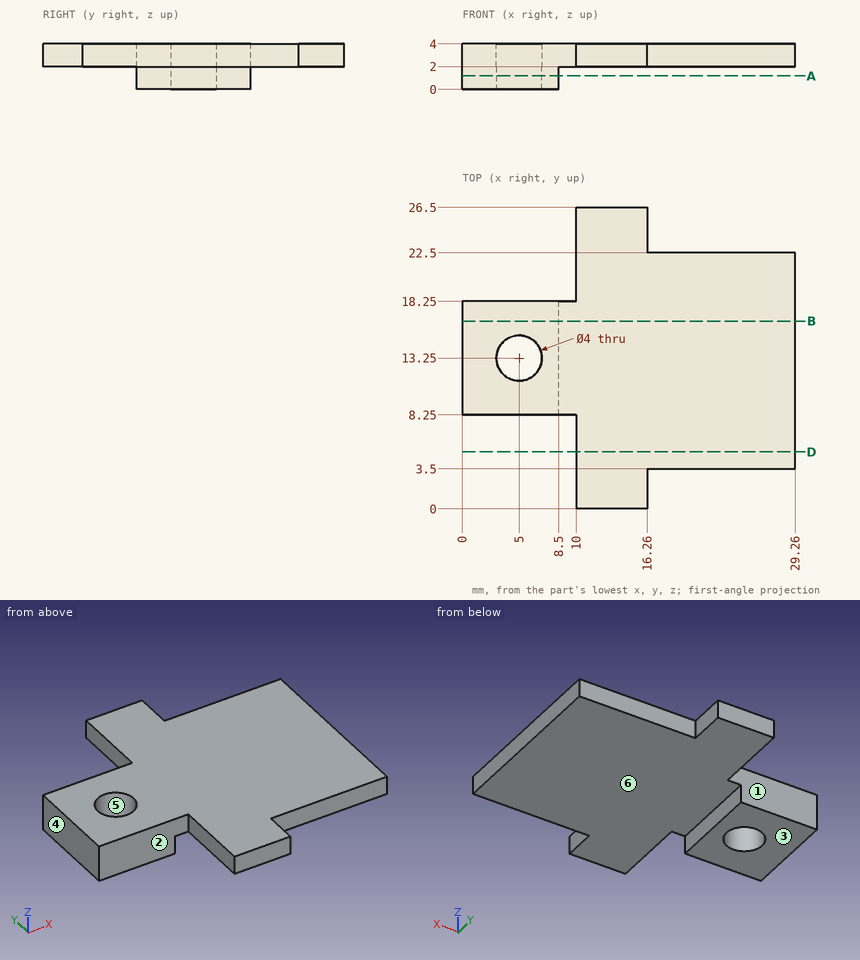
Print and shaded views of the part. All mm, measured from the part's lowest x, y and z. A direction names the side the tool comes from. Coordinates: 2 decimals unless noted, no trailing zeros. Loops run counter-clockwise (first coordinate to the right, second up) from the corner with the lowest first, then second, coordinate; pieces in that order, holes last. Notation, with made-up numbers: (39.25, -34.75) -> (88.25, -34.75) arc R25 cw to (88.25, -6.75) -> close; hole circle Ø2 at (19, 28). An arc over 180 degrees is marked (long way). Use one line per item in the form item = value. Start each with the question number.
(1) Flat gauge pins, fed straight in: pin 1 (1 mm diameter, centred on y = 21, z = 3, fed in from -X); pin 2 (1 mm diameter, centred on x = 11.5, y = 19, fed in from -Z); pin 3 (1 mm diameter, centred on y = 2, z = 3, fed in from +X). Where does each tip first touch, or does it go through?
(2) Cut at B-B on y = 16.5. Give the cut face in (x, z), and give its area (3 significant figures).
(3) Pull direction X, two halves, no side cores. Call the marked faces 4, 5 and 6: pulls with the +X half, pulls with the -X half, needs draft (parallel to the pull), parting line crosses it, or undercut.
(4) Cut at D-D on y = 5. Give the cut face in (x, z).
(5) Tool access for the marked faces 1, 2 and 3: list every direction of +Z, -Z, +X, -X, +Y, -Y with a clear straight run to the whole face (end or side of a thin tool).
(6) Cut at A-A on z = 1.2. Give the cut face in (x, y).
(7) Probe probe 1 along Y at (x, z) = (5, 3); probe 2 along X at (y, z) = (13.25, 1.5); probe 3 along X at (y, z) = (7, 3.6). List the from-to ranges inside material, lowest first. Write a range as from..to.
Values:
q1.pin_1 = 10
q1.pin_2 = 2
q1.pin_3 = 16.26
q2.outline = (0, 0) -> (8.5, 0) -> (8.5, 2) -> (29.26, 2) -> (29.26, 4) -> (0, 4) -> close
q2.area = 75.5 mm2
q3.face_4 = pulls with the -X half
q3.face_5 = undercut
q3.face_6 = needs draft
q4.outline = (10, 2) -> (29.26, 2) -> (29.26, 4) -> (10, 4) -> close
q5.face_1 = +Z, -Z, -X, +Y
q5.face_2 = +Z, -Z, -X, -Y
q5.face_3 = -Z, +X, -X, +Y, -Y
q6.outline = (0, 8.25) -> (8.5, 8.25) -> (8.5, 18.25) -> (0, 18.25) -> close; hole circle Ø4 at (5, 13.25)
q7.probe_1 = 8.25..11.25, 15.25..18.25
q7.probe_2 = 0..3, 7..8.5
q7.probe_3 = 10..29.26
